```python
from build123d import *

# Parameters (mm, degrees)
SKETCH1_R                                       = 2.6
BOSS_EXTRUDE1_DEPTH                             = 6
SKETCH2_R                                       = 3.25
BOSS_EXTRUDE2_DEPTH                             = 2
SKETCH3_R                                       = 2.5
BOSS_EXTRUDE3_DEPTH                             = 2.7
CSK_FOR_M5_FLAT_HEAD_MACHINE_SCREW1_D           = 5.5
CSK_FOR_M5_FLAT_HEAD_MACHINE_SCREW1_CSINK_D     = 10.4
CSK_FOR_M5_FLAT_HEAD_MACHINE_SCREW1_CSINK_ANGLE = 90
SKETCH7_R                                       = 2.6
BOSS_EXTRUDE5_DEPTH                             = 21
SKETCH8_W                                       = 43
SKETCH8_H                                       = 10
BOSS_EXTRUDE6_DEPTH                             = 50
SKETCH9_W                                       = 4.8
SKETCH9_H                                       = 10
SKETCH9_W_2                                     = 5.031184409
CUT_EXTRUDE1_DEPTH                              = 50


with BuildPart() as part:
    # Sketch1 → Boss-Extrude1 (new body)
    with BuildSketch(Plane(origin=(0, 0, 0), x_dir=(1, 0, 0), z_dir=(0, 1, 0))):
        with BuildLine():
            Line((5.031184409, -3), (0, -3))
            Line((0, -3), (0, -46))
            Line((0, -46), (50, -46))
            Line((50, -46), (50, -3))
            Line((50, -3), (44.968815591, -3))
            ThreePointArc((44.968815591, -3), (25, -7.79226602), (5.031184409, -3))
        make_face()
        with Locations(Location((15, -36, 0), (0, 0, 270))):
            Circle(SKETCH1_R, mode=Mode.SUBTRACT)
        with Locations(Location((35, -36, 0), (0, 0, 270))):
            Circle(SKETCH1_R, mode=Mode.SUBTRACT)
        with Locations(Location((15, -16, 0), (0, 0, 270))):
            Circle(SKETCH1_R, mode=Mode.SUBTRACT)
        with Locations(Location((35, -16, 0), (0, 0, 270))):
            Circle(SKETCH1_R, mode=Mode.SUBTRACT)
    extrude(amount=BOSS_EXTRUDE1_DEPTH)

    # Sketch2 → Boss-Extrude2 (add)
    with BuildSketch(Plane(origin=(0, 6, 0), x_dir=(1, 0, 0), z_dir=(0, 1, 0))):
        with Locations(Location((25, -17.5, 0), (0, 0, 270))):
            Circle(SKETCH2_R)
    extrude(amount=BOSS_EXTRUDE2_DEPTH)

    # Sketch3 → Boss-Extrude3 (add)
    with BuildSketch(Plane(origin=(0, 8, 0), x_dir=(1, 0, 0), z_dir=(0, 1, 0))):
        with Locations(Location((25, -17.5, 0), (0, 0, 90))):
            Circle(SKETCH3_R)
    extrude(amount=BOSS_EXTRUDE3_DEPTH)

    # CSK for M5 Flat Head Machine Screw1 (through all)
    with Locations(Plane(origin=(0, 6, 0), x_dir=(1, 0, 0), z_dir=(0, 1, 0))):
        with Locations((15, -16), (35, -16)):
            CounterSinkHole(CSK_FOR_M5_FLAT_HEAD_MACHINE_SCREW1_D / 2, CSK_FOR_M5_FLAT_HEAD_MACHINE_SCREW1_CSINK_D / 2, counter_sink_angle=CSK_FOR_M5_FLAT_HEAD_MACHINE_SCREW1_CSINK_ANGLE)

    # Sketch7 → Boss-Extrude5 (add)
    with BuildSketch(Plane(origin=(0, 6, 0), x_dir=(1, 0, 0), z_dir=(0, 1, 0))):
        with BuildLine():
            Line((21.039948447, -30.928253487), (0, -30.928253487))
            Line((0, -30.928253487), (0, -46))
            Line((0, -46), (50, -46))
            Line((50, -46), (50, -30.580877922))
            Line((50, -30.580877922), (29.989051292, -30.580877922))
            ThreePointArc((29.989051292, -30.580877922), (25.543026299, -31.489464694), (21.039948447, -30.928253487))
        make_face()
        with Locations(Location((15, -36, 0), (0, 0, 270))):
            Circle(SKETCH7_R, mode=Mode.SUBTRACT)
        with Locations(Location((35, -36, 0), (0, 0, 270))):
            Circle(SKETCH7_R, mode=Mode.SUBTRACT)
    extrude(amount=BOSS_EXTRUDE5_DEPTH)

    # Sketch8 → Boss-Extrude6 (add)
    with BuildSketch(Plane.ZY):
        with Locations((24.5, -5)):
            Rectangle(SKETCH8_W, SKETCH8_H)
    extrude(amount=-BOSS_EXTRUDE6_DEPTH)

    # Sketch9 → Cut-Extrude1 (cut)
    with BuildSketch(Plane(origin=(0, 0, 3), x_dir=(-1, 0, 0), z_dir=(0, 0, -1))):
        with Locations((-47.6, -5)):
            Rectangle(SKETCH9_W, SKETCH9_H)
        with Locations((-2.515592205, -5)):
            Rectangle(SKETCH9_W_2, SKETCH9_H)
    extrude(amount=-CUT_EXTRUDE1_DEPTH, mode=Mode.SUBTRACT)


solid = part.part
```
For this review, take the finished solid that the model builds, in its own axes (mm). A direction names the side the tool comes from. Round coordinates to 2 decimals unless told otherwise and drop trailing zeros. Write each loop counter-clockwise with the first axis right and the second up, starting at its lowest first coordinate (ties: lowest second). Pieces come first, ordered by that corner, then holes. Notation, with made-up numbers: (17.5, 10.5) -> (44.5, 10.5) arc R22 cw to (44.5, 42.5) -> close; hole circle Ø5 at (87.5, -8). An arc over 180 degrees is marked (long way). One line per question, with ' | ' between items. Start each with the question number.
(1) Add section D-D, the plane z = 36. Write out the cut boundary in (x, y), plus the area to 3 significant figures.
(2) Add section C-C, the plane x = 35. Write out the cut boundary in (y, z).
(3) Mouldability with a two-part tool opening along Z and no side actions: class faces 1 (the face through (25, 8, 46)), 2 (the face through (45.2, -5, 24)), 3 (the face through (11, 16, 30.928)), 4 (the face through (17.115, 3.669, 14.061)) as released by +Z, released by -Z, zero draft, split by the parting line, or undercut.
(4) Insertion check: P1, Ø2, axis at x = 15, z = 10, coming from the +Y side; P2, Ø4, axis at x = 24, z = 17.5, coming from the +Y side; P3, Ø5, axis at x = 25.5, y = 12, coming from the -Z side; P4, Ø12, axis at y = -5, z = 39.5, coming from the -X side. Each pin has a flat end and moves straight along its axis. Give the tip position at first contact, or say it passes through.
(5) Add section B-B, the plane z = 29.5. Write out the cut boundary in (x, y), plus the area to 3 significant figures.
(6) Tool access review of faces 5 (the face through (25.29, 2.96, 7.79)), 6 (the face through (2, 3, 3)), 7 (the face through (25, 10.7, 18)), 8 (the face through (17.747, 1.75, 15.879)): name each direction out of +Z, -Z, +X, -X, +Y, -Y from which nothing blocks a thin tool from reaching the whole face with its end or side.
(7) For line 1 along X through (y, z) = (13, 36); line 2 along X through (y, z) = (1, 16); line 3 along Z through (x, y) = (6, 15), list the stretches that pass through material, from the lowest coordinate up. Write a range as from..to.
(8) Add section A-A, the plane y = 17.5. Write out the cut boundary in (x, z), plus the area to 3 significant figures.
Answer list:
1) outline: (0, 0) -> (5.03, 0) -> (5.03, -10) -> (45.2, -10) -> (45.2, 0) -> (50, 0) -> (50, 27) -> (37.6, 27) -> (37.6, 0) -> (32.4, 0) -> (32.4, 27) -> (17.6, 27) -> (17.6, 0) -> (12.4, 0) -> (12.4, 27) -> (0, 27) -> close | area: 1,470 mm²
2) outline: (-10, 3) -> (0, 3) -> (0, 6.64) -> (6, 6.64) -> (6, 10.8) -> (3.55, 13.25) -> (0, 13.25) -> (0, 18.75) -> (3.55, 18.75) -> (6, 21.2) -> (6, 30.58) -> (27, 30.58) -> (27, 33.4) -> (0, 33.4) -> (0, 38.6) -> (27, 38.6) -> (27, 46) -> (-10, 46) -> close
3) face 1: released by +Z | face 2: zero draft | face 3: released by -Z | face 4: undercut
4) P1: y = 6 | P2: y = 10.7 | P3: z = 15 | P4: x = 0
5) outline: (0, 0) -> (5.03, 0) -> (5.03, -10) -> (45.2, -10) -> (45.2, 0) -> (50, 0) -> (50, 6) -> (0, 6) -> close | area: 702 mm²
6) face 5: -Z, +Y | face 6: -Z, +X, -X, +Y, -Y | face 7: -Z, +X, -X, +Y | face 8: +Y
7) line 1: 0..12.4, 17.6..32.4, 37.6..50 | line 2: 0..12.25, 17.75..32.25, 37.75..50 | line 3: 30.93..46
8) outline: (0, 30.93) -> (21.04, 30.93) arc R14 cw to (29.99, 30.58) -> (50, 30.58) -> (50, 46) -> (0, 46) -> close; hole circle Ø5.2 at (15, 36); hole circle Ø5.2 at (35, 36) | area: 715 mm²
